```python
from build123d import *

# Parameters (mm, degrees)
F0_R     = 40
F1_DEPTH = 80
F2_R     = 10
F3_T     = -2
F4_W     = 75
F4_H     = 45
F5_DEPTH = 7.5
F6_R     = 15


with BuildPart() as f1:
    # F0 (on Top) → F1 (new body)
    with BuildSketch(Plane.XY):
        Circle(F0_R)
    extrude(amount=F1_DEPTH)

    # F2
    f2_edges = [f1.edges().sort_by_distance(p)[0] for p in [
        (-40, 0, 0),
    ]]
    fillet(f2_edges, radius=F2_R)

    # F3
    f3_openings = [f1.faces().sort_by_distance(p)[0] for p in [
        (0, 0, 80),
    ]]
    offset(amount=F3_T, openings=f3_openings)

    # F4 (on Front) → F5 (join, symmetric)
    with BuildSketch(Plane.XZ):
        with Locations((37.5, 42.5)):
            Rectangle(F4_W, F4_H)
    extrude(amount=F5_DEPTH, both=True)

    # F6
    f6_edges = [f1.edges().sort_by_distance(p)[0] for p in [
        (75, 0, 65),
        (75, 0, 20),
    ]]
    fillet(f6_edges, radius=F6_R)


solid = f1.part
```
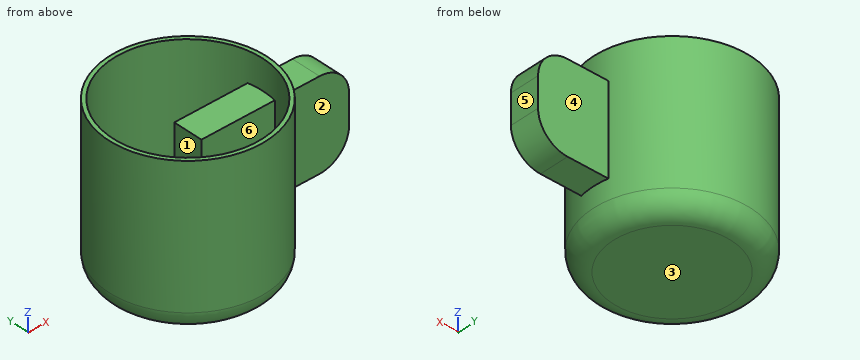
Check sheet for the modelled part. Datum: model origin and axes. Units: mm. Face numbers are marked on the shaded views. A direction names the side the tool comes from. Give positions to 0.01 mm unless a question says otherwise; leave off trailing zeros. Loops run counter-clockwise (first coordinate to the right, second up) from the corner with the lowest first, then second, coordinate; pieces in that order, holes last. Notation, with made-up numbers: M 51,80.25 L 103,80.25 A9 ccw 103,87.25 Z; hole C 82.25,-2.75 d7. An arc over 180 degrees is marked long. Answer as CSV lines item,"result".
Item 1: Sectioned sample at A-A, the plane z = 42. Enter the section's corners in (x, y), then the cut area to 3 significant figures.
Reply:
outline,"M 39.29,-7.5 L 75,-7.5 L 75,7.5 L 39.29,7.5 A40 ccw long Z; hole M 0,-7.5 L 0,7.5 L 37.25,7.5 A38 ccw long 37.25,-7.5 Z"
area,"1,580 mm^2"
Item 2: Scan lines: L1, parallel to Y at x = 23.5, z = 36; L2, parallel to Y at x = 12, z = 30; L3, parallel to X at y = -2.5, z = 69.5. Record each from-to range of solid material in increasing order.
Reply:
L1,"-32.37 to -29.86, -7.5 to 7.5, 29.86 to 32.37"
L2,"-38.16 to -36.06, -7.5 to 7.5, 36.06 to 38.16"
L3,"-39.92 to -37.92, 37.92 to 39.92"
Item 3: Draft check along X on the marked faces 4, 5 and 6. Enter one of: pulls with the +X half, pulls with the -X half, needs draft (parallel to the pull), parting line crosses it, or undercut.
Reply:
face 4,"needs draft"
face 5,"pulls with the +X half"
face 6,"undercut"
Item 4: Sectioned sample at B-B, the plane y = 0. Enter the section's corners in (x, z).
Reply:
outline,"M -40,10 A10 ccw -30,0 L 30,0 A10 ccw 40,10 L 40,20 L 60,20 A15 ccw 75,35 L 75,50 A15 ccw 60,65 L 40,65 L 40,80 L 38,80 L 38,65 L 0,65 L 0,20 L 38,20 L 38,10 A8 cw 30,2 L -30,2 A8 cw -38,10 L -38,80 L -40,80 Z"
Item 5: Sectioned sample at C-C, the plane z = 70.5. Enter the section's corners in (x, y), then the cut area to 3 significant figures.
Reply:
outline,"C 0,0 d80; hole C 0,0 d76"
area,"490 mm^2"
Item 6: Depth check by flat-ended pin: pin 1 Ø8 at (x, y) = (16, 16.5) entering from +Z; pin 2 Ø16.5 at (x, y) = (24, 2.5) entering from -Z; pin 3 Ø7.5 at (x, y) = (12.5, 1.5) entering from +Z; pin 4 Ø12 at (x, y) = (53, 3.5) entering from -Z. Enter the tip coordinate at first touch or a pass-through.
Reply:
pin 1,"z = 2"
pin 2,"z = 0"
pin 3,"z = 65"
pin 4,"z = 20"
Item 7: Set-up check for the marked faces 1, 2 and 3: record each of +Z, -Z, +X, -X, +Y, -Y from which the full face is reachable in a straight line by a thin tool's end or side.
Reply:
face 1,"+Z"
face 2,"+Z, -Z, +X, -Y"
face 3,"-Z, +X, -X, +Y, -Y"
